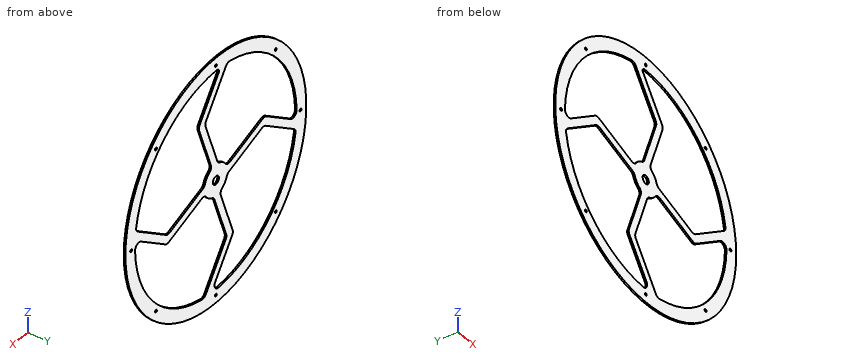
```python
from build123d import *

# Parameters (mm, degrees)
F0_R     = 235
F0_R_2   = 2.5
F0_R_3   = 8
F1_DEPTH = 3


with BuildPart() as f1:
    # F0 (on Front) → F1 (new body)
    with BuildSketch(Plane.XZ):
        Circle(F0_R)
        with Locations((-155.563492, -155.563492)):
            Circle(F0_R_2, mode=Mode.SUBTRACT)
        with BuildLine():
            ThreePointArc((-129.064274, 25.601808), (-124.657231, 27.32162), (-119.952823, 26.823297))
            Line((-119.952823, 26.823297), (-34.352843, -3.874505))
            ThreePointArc((-34.352843, -3.874505), (-30.637301, -6.236665), (-28.296397, -9.965636))
            ThreePointArc((-28.296397, -9.965636), (-23.711827, -18.377956), (-16.709034, -24.916022))
            ThreePointArc((-16.709034, -24.916022), (-12.779669, -30.095956), (-12.865703, -36.59705))
            Line((-12.865703, -36.59705), (-43.563506, -122.197029))
            ThreePointArc((-43.563506, -122.197029), (-44.061828, -126.901437), (-42.342017, -131.30848))
            Line((-42.342017, -131.30848), (1.665505, -194.157735))
            ThreePointArc((1.665505, -194.157735), (2.267567, -204.655106), (-6.852316, -209.888174))
            ThreePointArc((-6.852316, -209.888174), (-137.800831, -158.464289), (-206.904803, -35.922171))
            ThreePointArc((-206.904803, -35.922171), (-206.28595, -30.372613), (-202.787958, -26.020071))
            Line((-202.787958, -26.020071), (-129.064274, 25.601808))
        make_face(mode=Mode.SUBTRACT)
        with Locations((0, -220)):
            Circle(F0_R_2, mode=Mode.SUBTRACT)
        with Locations((155.563492, -155.563492)):
            Circle(F0_R_2, mode=Mode.SUBTRACT)
        with BuildLine():
            ThreePointArc((24.916022, -16.709034), (30.095956, -12.779669), (36.59705, -12.865703))
            Line((36.59705, -12.865703), (122.197029, -43.563506))
            ThreePointArc((122.197029, -43.563506), (126.901437, -44.061828), (131.30848, -42.342017))
            Line((131.30848, -42.342017), (194.157735, 1.665505))
            ThreePointArc((194.157735, 1.665505), (204.655106, 2.267567), (209.888174, -6.852316))
            ThreePointArc((209.888174, -6.852316), (158.464289, -137.800831), (35.922171, -206.904803))
            ThreePointArc((35.922171, -206.904803), (30.372613, -206.28595), (26.020071, -202.787958))
            Line((26.020071, -202.787958), (-25.601808, -129.064274))
            ThreePointArc((-25.601808, -129.064274), (-27.32162, -124.657231), (-26.823297, -119.952823))
            Line((-26.823297, -119.952823), (3.874505, -34.352843))
            ThreePointArc((3.874505, -34.352843), (6.236665, -30.637301), (9.965636, -28.296397))
            ThreePointArc((9.965636, -28.296397), (18.377956, -23.711827), (24.916022, -16.709034))
        make_face(mode=Mode.SUBTRACT)
        with Locations((-220, 0)):
            Circle(F0_R_2, mode=Mode.SUBTRACT)
        with BuildLine():
            ThreePointArc((-3.874505, 34.352843), (-6.236665, 30.637301), (-9.965636, 28.296397))
            ThreePointArc((-9.965636, 28.296397), (-18.377956, 23.711827), (-24.916022, 16.709034))
            ThreePointArc((-24.916022, 16.709034), (-30.095956, 12.779669), (-36.59705, 12.865703))
            Line((-36.59705, 12.865703), (-122.197029, 43.563506))
            ThreePointArc((-122.197029, 43.563506), (-126.901437, 44.061828), (-131.30848, 42.342017))
            Line((-131.30848, 42.342017), (-194.157735, -1.665505))
            ThreePointArc((-194.157735, -1.665505), (-204.655106, -2.267567), (-209.888174, 6.852316))
            ThreePointArc((-209.888174, 6.852316), (-158.464289, 137.800831), (-35.922171, 206.904803))
            ThreePointArc((-35.922171, 206.904803), (-30.372613, 206.28595), (-26.020071, 202.787958))
            Line((-26.020071, 202.787958), (25.601808, 129.064274))
            ThreePointArc((25.601808, 129.064274), (27.32162, 124.657231), (26.823297, 119.952823))
            Line((26.823297, 119.952823), (-3.874505, 34.352843))
        make_face(mode=Mode.SUBTRACT)
        with Locations((-155.563492, 155.563492)):
            Circle(F0_R_2, mode=Mode.SUBTRACT)
        Circle(F0_R_3, mode=Mode.SUBTRACT)
        with BuildLine():
            ThreePointArc((-3.213168, 209.975417), (133.963441, 161.721354), (206.904803, 35.922171))
            ThreePointArc((206.904803, 35.922171), (206.28595, 30.372613), (202.787958, 26.020071))
            Line((202.787958, 26.020071), (129.064274, -25.601808))
            ThreePointArc((129.064274, -25.601808), (124.657231, -27.32162), (119.952823, -26.823297))
            Line((119.952823, -26.823297), (34.352843, 3.874505))
            ThreePointArc((34.352843, 3.874505), (30.637301, 6.236665), (28.296397, 9.965636))
            ThreePointArc((28.296397, 9.965636), (23.711827, 18.377956), (16.709034, 24.916022))
            ThreePointArc((16.709034, 24.916022), (12.779669, 30.095956), (12.865703, 36.59705))
            Line((12.865703, 36.59705), (43.563506, 122.197029))
            ThreePointArc((43.563506, 122.197029), (44.061828, 126.901437), (42.342017, 131.30848))
            Line((42.342017, 131.30848), (-7.232424, 202.10812))
            ThreePointArc((-7.232424, 202.10812), (-7.589252, 207.250746), (-3.213168, 209.975417))
        make_face(mode=Mode.SUBTRACT)
        with Locations((220, 0)):
            Circle(F0_R_2, mode=Mode.SUBTRACT)
        with Locations((0, 220)):
            Circle(F0_R_2, mode=Mode.SUBTRACT)
        with Locations((155.563492, 155.563492)):
            Circle(F0_R_2, mode=Mode.SUBTRACT)
    extrude(amount=F1_DEPTH)


solid = f1.part
```
CAD build for the part. Positions are in the model's coordinates, mm. Round coordinates to 2 decimals unless told otherwise and drop trailing zeros. Order: outer loops, then holes, each group sorted by start corner. A loop starts at its lowest first (then second) coordinate and runs counter-clockwise, first axis right, second up.
Item 1: Saw through at A-A on z = -93.5. Write the cut outline in (x, y), then the cut area to 3 significant figures.
Item 2: Pin check, flat tips, straight feed: pin 1 (1.5 mm diameter, centred on x = -103, y = -1, fed in from -Z); pin 2 (6 mm diameter, centred on x = -220, z = 0, fed in from -Y). Stop position of each tip, or through.
Item 3: Probe line 1 along X through (y, z) = (-2.5, -188.5); line 2 along X through (y, z) = (-0.5, 45); line 3 along Z through (x, y) = (126.5, -1.6). List the from-to ranges inside material, lowest first.
Item 4: Saw through at C-C on y = -2.1. State how many separate pieces and enclosed holes the cut face has, then the cut area to 3 significant figures.
Item 5: Saw through at B-B on z = 181.5. Write the cut outline in (x, y).
Reported:
1. outline: (-215.6, -3) - (-188.04, -3) - (-188.04, 0) - (-215.6, 0) - close; (-33.27, -3) - (-17.34, -3) - (-17.34, 0) - (-33.27, 0) - close; (188.04, -3) - (215.6, -3) - (215.6, 0) - (188.04, 0) - close
1. area: 213 mm2
2. pin 1: stops at z = -211.59
2. pin 2: stops at y = -3
3. line 1: x = -140.33 to -92.56, -2.3 to 16.02, 92.56 to 140.33
3. line 2: x = -230.65 to -205.12, -0.06 to 15.88, 205.12 to 230.65
3. line 3: z = -198.05 to -167.62, -44.11 to -26.89, 167.62 to 198.05
4. separate pieces: 1
4. enclosed holes: 13
4. area: 50,000 mm2
5. outline: (-149.27, -3) - (-105.63, -3) - (-105.63, 0) - (-149.27, 0) - close; (-11.11, -3) - (7.2, -3) - (7.2, 0) - (-11.11, 0) - close; (105.63, -3) - (149.27, -3) - (149.27, 0) - (105.63, 0) - close
